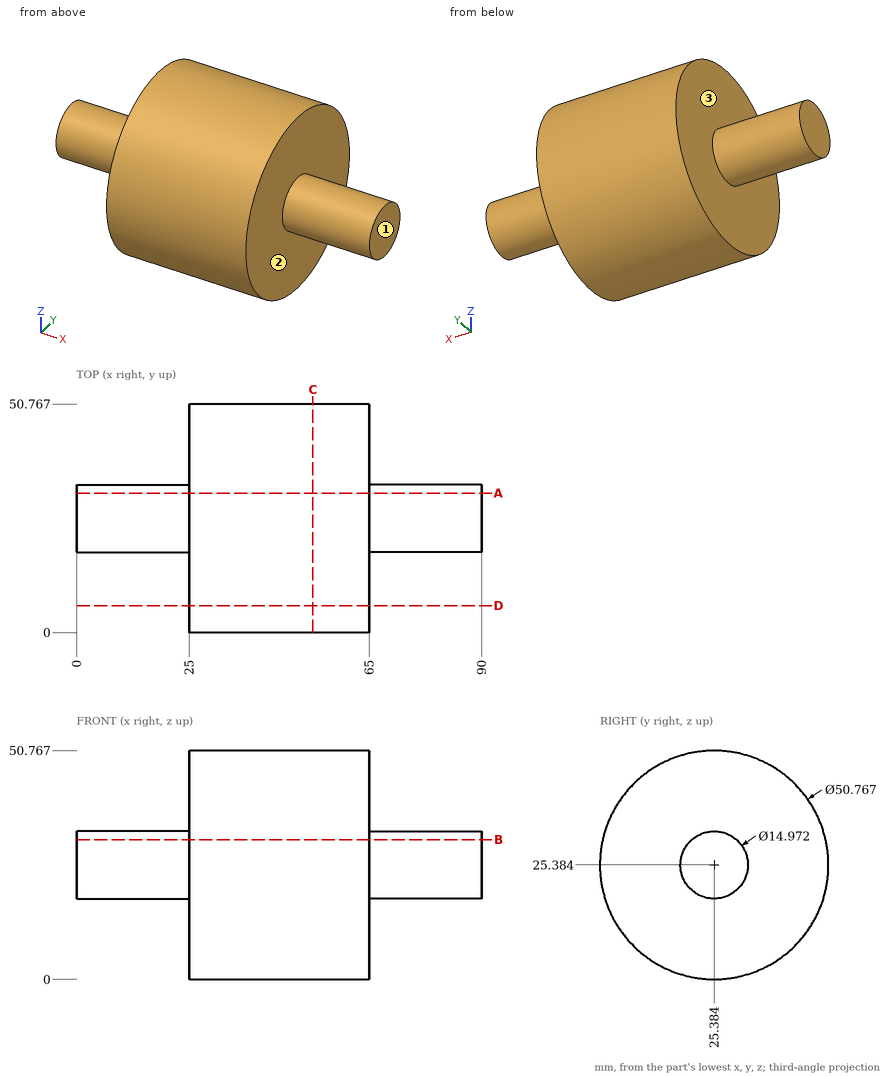
Print and shaded views of the part. All mm, measured from the part's lowest x, y and z. A direction names the side the tool comes from. Coordinates: 2 decimals unless noted, no trailing zeros. Loops run counter-clockwise (first coordinate to the right, second up) from the corner with the lowest first, then second, coordinate; pieces in that order, holes last. Notation, with made-up numbers: (68.25, 40.5) - (101.25, 40.5) arc R16 cw to (101.25, 44.5) - close; hole circle Ø4 at (81, -20.75). An arc over 180 degrees is marked (long way). Write item = value, one per line. Start each with the question number.
Item 1: Cut at D-D, the plane y = 6. Give the cut face in (x, z) (1 decimal), and give its area (3 significant figures).
Item 2: Wall check: L1, parallel to X at y = 10, z = 33; L2, parallel to Z at x = 58.5, y = 24.5 (1 decimal); L3, parallel to Y at x = 61, z = 25.5. Give the ranges that are in metal, low to high. Write a range as from..to.
Item 3: Flat gauge pins, fed straight in: pin 1 Ø4 at (x, y) = (35.5, 31) entering from +Z; pin 2 Ø4 at (x, z) = (64, 36.5) entering from -Y; pin 3 Ø4 at (x, y) = (41, 15) entering from +Z. Where does each tip first touch, or does it go through?
Item 4: Cut at A-A, the plane y = 31. Give the cut face in (x, z) (1 decimal).
Item 5: Cut at C-C, the plane x = 52.5. Give the cut face in (y, z), and give its area (3 significant figures).
Item 6: 3-axis set-ups, long thin cutter, end or side, ignore diameter. For the marked faces 1, 2 and 3: which of +Z, -Z, +X, -X, +Y, -Y reach the whole face in a straight line?
The answers:
q1.outline = (25, 9) - (65, 9) - (65, 41.8) - (25, 41.8) - close
q1.area = 1,310 mm2
q2.L1 = 25..65
q2.L2 = 0..50.8
q2.L3 = 0..50.77
q3.pin_1 = 50.51
q3.pin_2 = 1.69
q3.pin_3 = 49.34
q4.outline = (0, 20.4) - (25, 20.4) - (25, 0.6) - (65, 0.6) - (65, 20.4) - (90, 20.4) - (90, 30.3) - (65, 30.3) - (65, 50.1) - (25, 50.1) - (25, 30.3) - (0, 30.3) - close
q5.outline = circle Ø50.77 at (25.38, 25.38)
q5.area = 2,020 mm2
q6.face_1 = +Z, -Z, +X, +Y, -Y
q6.face_2 = +X
q6.face_3 = -X
